Can you work these out from the drawing? Everything is in mm from the part's minimum corner. A direction names the side the tool comes from. Coordinates: 2 decimals unless noted, no trailing zeros. Write each loop counter-clockwise with the first axis right and the second up, starting at its lowest first coordinate (ties: lowest second). Pieces come first, ordered by that corner, then holes.
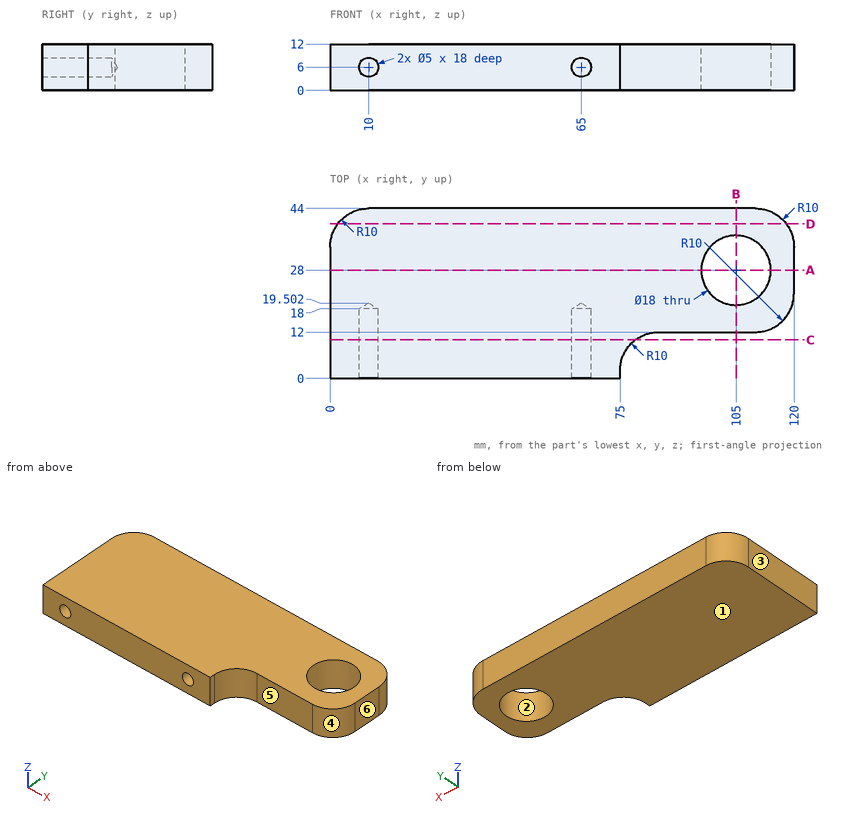
1. On a 3-axis mill with a long thin cutter (end or side, diameter ignored), from which of +Z, -Z, +X, -X, +Y, -Y can I reach the whole of each face in a straight line? I mean the marked faces 5 and 6. Say none if no direction works.
2. I want a section at C-C (y = 10). List the corners of the cut face in (x, z) for me.
3. I want a section at D-D (y = 40). List the corners of the cut face in (x, z) for me, then the cut area to 3 significant figures.
4. I want a section at A-A (y = 28). List the corners of the cut face in (x, z) for me.
5. For pin 1 Ø2 at (y, z) = (1, 4) entering from +X; pin 2 Ø6 at (x, y) = (45, 17) entering from -Z, each with a flat end and sliding along its axis, tell me the tip position at first contact or that it passes through.
6. I want a section at B-B (x = 105). List the corners of the cut face in (y, z) for me, then the cut area to 3 significant figures.
7. If I drill on line 1 (X direction, y = 8.5, z = 8); line 2 (Z direction, x = 65, y = 8.25); line 3 (X direction, y = 29, z = 9.25), over which ranges is the centre line in solid material (lowest first)?
8. Thinking about a two-plate mould opening in X: for the marked faces 1, 2, 3 and 4, which applies, pulls with the +X half, pulls with the -X half, needs draft (parallel to the pull), parting line crosses it, or undercut?
Response values:
1. face 5: +Z, -Z, +X, -Y
1. face 6: +Z, -Z, +X, +Y, -Y
2. outline: (0, 0) - (79, 0) - (79, 12) - (0, 12) - close; hole circle Ø5 at (10, 6); hole circle Ø5 at (65, 6)
3. outline: (2, 0) - (118, 0) - (118, 12) - (2, 12) - close
3. area: 1,390 mm2
4. outline: (0, 0) - (96, 0) - (96, 12) - (0, 12) - close; (114, 0) - (120, 0) - (120, 12) - (114, 12) - close
5. pin 1: stops at x = 75
5. pin 2: stops at z = 0
6. outline: (12, 0) - (19, 0) - (19, 12) - (12, 12) - close; (37, 0) - (44, 0) - (44, 12) - (37, 12) - close
6. area: 168 mm2
7. line 1: x = 0 to 8.5, 11.5 to 63.5, 66.5 to 77.4
7. line 2: z = 0 to 3.5, 8.5 to 12
7. line 3: x = 0 to 96.06, 113.94 to 120
8. face 1: needs draft
8. face 2: undercut
8. face 3: pulls with the -X half
8. face 4: pulls with the +X half
